from build123d import *

# Parameters (mm, degrees)
F1_DEPTH = 22.86
F2_R     = 11.43
F3_DEPTH = 22.861
F5_DEPTH = 22.225
F7_DEPTH = 11.9126


with BuildPart() as f1:
    # F0 (on Top) → F1 (new body)
    with BuildSketch(Plane.XY):
        Polygon((-16.51, 18.415), (-16.51, 0), (-16.51, -18.415), (16.51, -18.415), (16.51, 18.415), align=None)
    extrude(amount=F1_DEPTH)

    # F2 (on Top) → F3 (cut, through all)
    with BuildSketch(Plane.XY):
        Circle(F2_R)
    extrude(amount=F3_DEPTH, mode=Mode.SUBTRACT)

    # F4 (on Top) → F5 (cut)
    with BuildSketch(Plane.XY):
        Polygon((-15.24, 17.78), (-15.24, 0), (-15.24, -17.78), (-15.24, -25.4), (15.24, -25.4), (15.24, -17.78), (15.24, 17.78), align=None)
    extrude(amount=F5_DEPTH, mode=Mode.SUBTRACT)

    # F6 (on Top) → F7 (cut)
    with BuildSketch(Plane.XY):
        Polygon((12.568022, 0), (0, 0), (-12.568022, 0), (-12.568022, -23.286249), (12.568022, -23.286249), align=None)
    extrude(amount=F7_DEPTH, mode=Mode.SUBTRACT)


solid = f1.part
Can you work these out from the model? Positions are in its coordinate system, mm. A direction names the side the tool comes from. Coordinates: 2 decimals unless noted, no trailing zeros. Write each loop counter-clockwise with the first axis right and the second up, starting at its lowest first coordinate (ties: lowest second). Pieces come first, ordered by that corner, then holes. Notation, with made-up numbers: (20.25, 65) -> (31.25, 65) arc R15 ccw to (31.25, 74) -> close; hole circle Ø9 at (11.5, 51). An arc over 180 degrees is marked (long way). Write each question's results on one line, items separated by ' | '. Start each with the question number.
Q1. If I drill on probe 1 along X at (y, z) = (0, 22.75); probe 2 along X at (y, z) = (-7.5, 17.5); probe 3 along Y at (x, z) = (0, 22.5) (3 decimals), over which ranges is the centre line in solid material (lowest first)?
Q2. Imagine slicing it at D-D (x = -8). Write out the boundary of the cut face in (y, z) (3 decimals), then the cut area to 3 significant figures.
Q3. Imagine slicing it at B-B (y = 0). Write out the boundary of the cut face in (x, z) (3 decimals), then the cut area to 3 significant figures.
Q4. Imagine slicing it at A-A (x = 0). Write out the boundary of the cut face in (y, z) (3 decimals), then the cut area to 3 significant figures.
Q5. I'm going to push flat-ended pins straight in: pin 1 (3 mm diameter, centred on x = -11.5, y = 12.5, fed in from -Z) (3 decimals); pin 2 (6.5 mm diameter, centred on x = 3, z = 10, fed in from -Y). Where does each tip first touch, or does it pass through?
Q6. On a 3-axis mill with a long thin cutter (end or side, diameter ignored), from which of +Z, -Z, +X, -X, +Y, -Y can I reach the whole of each face in a straight line? I mean faces 1 (the face through (-0.1, -18.415, 22.4)), 2 (the face through (0, 12, 22.225)). Say none if no direction works.
Q7. We'd pull the mould along X, two halves only. Please class faces 3 (the face through (0, 18.415, 11)), 4 (the face through (15.24, -1, 11)), 5 (the face through (-16.51, 0, 11)): +X half, -X half, draft (parallel to the pull), parting line (faces both ways), or undercut.
Q8. Imagine slicing it at C-C (z = 12.25). Write out the boundary of the cut face in (x, y) (3 decimals).
Taken from the geometry:
1) probe 1: x = -16.51 to -11.43, 11.43 to 16.51 | probe 2: x = -16.51 to -15.24, 15.24 to 16.51 | probe 3: y = -18.415 to -11.43, 11.43 to 18.415
2) outline: (-18.415, 22.225) -> (-8.164, 22.225) -> (-8.164, 22.86) -> (-18.415, 22.86) -> close; (8.164, 22.225) -> (17.78, 22.225) -> (17.78, 0) -> (18.415, 0) -> (18.415, 22.86) -> (8.164, 22.86) -> close | area: 27.1 mm^2
3) outline: (-16.51, 0) -> (-15.24, 0) -> (-15.24, 22.225) -> (-11.43, 22.225) -> (-11.43, 22.86) -> (-16.51, 22.86) -> close; (11.43, 22.225) -> (15.24, 22.225) -> (15.24, 0) -> (16.51, 0) -> (16.51, 22.86) -> (11.43, 22.86) -> close | area: 62.9 mm^2
4) outline: (-18.415, 22.225) -> (-11.43, 22.225) -> (-11.43, 22.86) -> (-18.415, 22.86) -> close; (11.43, 22.225) -> (17.78, 22.225) -> (17.78, 0) -> (18.415, 0) -> (18.415, 22.86) -> (11.43, 22.86) -> close | area: 23.0 mm^2
5) pin 1: stops at z = 22.225 | pin 2: stops at y = 17.78
6) face 1: +Z, -Z, +X, -X, -Y | face 2: -Z, -Y
7) face 3: draft | face 4: undercut | face 5: -X half
8) outline: (-16.51, -18.415) -> (-15.24, -18.415) -> (-15.24, 17.78) -> (15.24, 17.78) -> (15.24, -18.415) -> (16.51, -18.415) -> (16.51, 18.415) -> (-16.51, 18.415) -> close
